Here's how the part is built. I have some questions about the finished solid (model axes, mm). Face numbers are marked on the shaded views. A direction names the side the tool comes from. Give positions to 0.01 mm unless a question says otherwise; leave off trailing zeros. Loops run counter-clockwise (first coordinate to the right, second up) from the corner with the lowest first, then second, coordinate; pieces in that order, holes last. Notation, with made-up numbers: (-11.5, 54.5) - (20.5, 54.5) arc R19 ccw to (20.5, 91.5) - close; hole circle Ø9 at (21.25, 64). An arc over 180 degrees is marked (long way). Use a Markdown table: item, result.
from build123d import *

# Parameters (mm, degrees)
F1_DEPTH      = 125
F3_DEPTH      = 5
F3_DEPTH_BACK = 10
F5_DEPTH      = 75


with BuildPart() as f1:
    # F0 (on Front) → F1 (new body)
    with BuildSketch(Plane.XZ):
        with BuildLine():
            Line((-37.5, 0), (-37.5, -40))
            Line((-37.5, -40), (37.5, -40))
            Line((37.5, -40), (37.5, 0))
            ThreePointArc((37.5, 0), (0, 37.5), (-37.5, 0))
        make_face()
    extrude(amount=F1_DEPTH)

    # F2 (on face) → F3 (join, two sides)
    with BuildSketch(Plane(origin=(0, 0, -40), x_dir=(1, 0, 0), z_dir=(0, 0, -1))) as f3_sk:
        with BuildLine():
            Line((52.5, 106), (52.5, 110))
            Line((52.5, 110), (-52.5, 110))
            Line((-52.5, 110), (-52.5, 106))
            ThreePointArc((-52.5, 106), (-47.550253, 103.949747), (-45.5, 99))
            ThreePointArc((-45.5, 99), (-47.550253, 94.050253), (-52.5, 92))
            Line((-52.5, 92), (-52.5, 88))
            Line((-52.5, 88), (-52.5, 32))
            Line((-52.5, 32), (-52.5, 28))
            ThreePointArc((-52.5, 28), (-47.550253, 25.949747), (-45.5, 21))
            ThreePointArc((-45.5, 21), (-47.550253, 16.050253), (-52.5, 14))
            Line((-52.5, 14), (-52.5, 10))
            Line((-52.5, 10), (52.5, 10))
            Line((52.5, 10), (52.5, 14))
            ThreePointArc((52.5, 14), (45.5, 21), (52.5, 28))
            Line((52.5, 28), (52.5, 32))
            Line((52.5, 32), (52.5, 88))
            Line((52.5, 88), (52.5, 92))
            ThreePointArc((52.5, 92), (45.5, 99), (52.5, 106))
        make_face()
        with BuildLine():
            ThreePointArc((52.5, 88), (63.5, 99), (52.5, 110))
            Line((52.5, 110), (52.5, 106))
            ThreePointArc((52.5, 106), (57.449747, 103.949747), (59.5, 99))
            ThreePointArc((59.5, 99), (57.449747, 94.050253), (52.5, 92))
            Line((52.5, 92), (52.5, 88))
        make_face()
        with BuildLine():
            Line((-52.5, 106), (-52.5, 110))
            ThreePointArc((-52.5, 110), (-63.5, 99), (-52.5, 88))
            Line((-52.5, 88), (-52.5, 92))
            ThreePointArc((-52.5, 92), (-59.5, 99), (-52.5, 106))
        make_face()
        with BuildLine():
            ThreePointArc((52.5, 10), (63.5, 21), (52.5, 32))
            Line((52.5, 32), (52.5, 28))
            ThreePointArc((52.5, 28), (57.449747, 25.949747), (59.5, 21))
            ThreePointArc((59.5, 21), (57.449747, 16.050253), (52.5, 14))
            Line((52.5, 14), (52.5, 10))
        make_face()
        with BuildLine():
            Line((-52.5, 28), (-52.5, 32))
            ThreePointArc((-52.5, 32), (-63.5, 21), (-52.5, 10))
            Line((-52.5, 10), (-52.5, 14))
            ThreePointArc((-52.5, 14), (-59.5, 21), (-52.5, 28))
        make_face()
    extrude(amount=F3_DEPTH)
    extrude(f3_sk.sketch, amount=-F3_DEPTH_BACK)

    # F4 (on Top) → F5 (join)
    with BuildSketch(Plane.XY):
        with BuildLine():
            Line((-24.016134, -56.944444), (-12.008067, -98.472222))
            ThreePointArc((-12.008067, -98.472222), (0, -107.5), (12.008067, -98.472222))
            Line((12.008067, -98.472222), (24.016134, -56.944444))
            ThreePointArc((24.016134, -56.944444), (0, -25), (-24.016134, -56.944444))
        make_face()
    extrude(amount=F5_DEPTH)


solid = f1.part
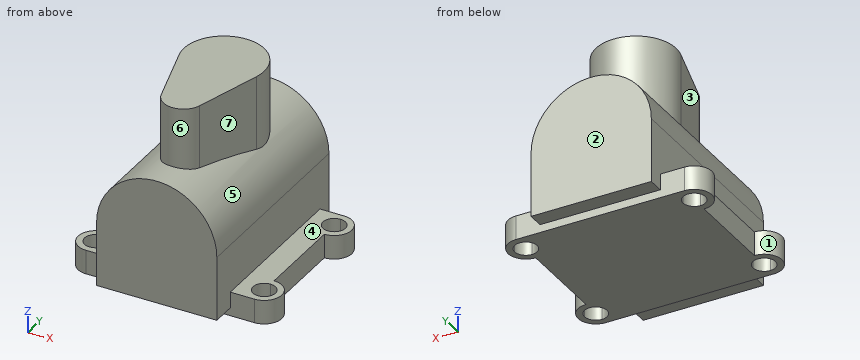
(1) Will these pins go through, and if not, where does the flat tip stop? pin 1 (4.5 mm diameter, centred on y = -71.5, z = -34.5, fed in from -X); pin 2 (5 mm diameter, centred on x = -13.5, y = -3, fed in from -Z); pin 3 (1.5 mm diameter, centred on y = -21.5, z = -25, fed in from +X).
A:
| item | result |
|---|---|
| pin 1 | x = -52.5 |
| pin 2 | z = -40 |
| pin 3 | x = 37.5 |
(2) Suppose I cut it at D-D on z = -12.5. Write out the boundary of the cut face in (x, y).
A:
| item | result |
|---|---|
| outline | (-37.5, -125) - (37.5, -125) - (37.5, 0) - (-37.5, 0) - close |
(3) Suppose I cut it at B-B on y = -103.5. Write out the boundary of the cut face in (x, z), plus the area to 3 significant figures.
A:
| item | result |
|---|---|
| outline | (-62.54, -45) - (-57.86, -45) - (-57.86, -30) - (-62.54, -30) - close; (-47.14, -45) - (47.14, -45) - (47.14, -30) - (37.5, -30) - (37.5, 0) arc R37.5 ccw to (9.17, 36.36) - (9.17, 75) - (-9.17, 75) - (-9.17, 36.36) arc R37.5 ccw to (-37.5, 0) - (-37.5, -30) - (-47.14, -30) - close; (57.86, -45) - (62.54, -45) - (62.54, -30) - (57.86, -30) - close |
| area | 6,710 mm2 |
(4) On a 3-axis mill with a long thin cutter (end or side, diameter ignored), from which of +Z, -Z, +X, -X, +Y, -Y can I reach the whole of each face in a straight line? I mean the marked faces 4, 5, 6 and 7. Say none if no direction works.
A:
| item | result |
|---|---|
| face 4 | +Z, +X, +Y, -Y |
| face 5 | +Z |
| face 6 | +Z, -Y |
| face 7 | +Z, +X, -Y |
(5) Suppose I cut it at A-A on x = 0. Write out the boundary of the cut face in (y, z), plus the area to 3 significant figures.
A:
| item | result |
|---|---|
| outline | (-125, -40) - (-110, -40) - (-110, -45) - (-10, -45) - (-10, -40) - (0, -40) - (0, 37.5) - (-25, 37.5) - (-25, 75) - (-107.5, 75) - (-107.5, 37.5) - (-125, 37.5) - close |
| area | 13,300 mm2 |
(6) If I drill on line 1 (Z direction, x = 41, y = -20); line 2 (X direction, y = -107, z = -25); line 3 (Z direction, x = -25, y = -32), over which ranges is the centre line in solid material (lowest first)?
A:
| item | result |
|---|---|
| line 1 | -45 to -30 |
| line 2 | -37.5 to 37.5 |
| line 3 | -45 to 27.95 |
(7) We'd pull the mould along Y, two halves only. Please class the marked faces 1, 2 and 3: pulls with the +Y half, pulls with the -Y half, needs draft (parallel to the pull), parting line crosses it, or undercut.
A:
| item | result |
|---|---|
| face 1 | undercut |
| face 2 | pulls with the +Y half |
| face 3 | pulls with the -Y half |
(8) Suppose I cut it at C-C on y = -50. Write out the boundary of the cut face in (x, z).
A:
| item | result |
|---|---|
| outline | (-52.5, -45) - (52.5, -45) - (52.5, -30) - (37.5, -30) - (37.5, 0) arc R37.5 ccw to (25, 27.95) - (25, 75) - (-25, 75) - (-25, 27.95) arc R37.5 ccw to (-37.5, 0) - (-37.5, -30) - (-52.5, -30) - close |
